Check sheet for the drawn part. Datum: minimum x, y, z corner. Units: mm. A direction names the side the tool comes from. Round coordinates to 2 decimals unless told otherwise and drop trailing zeros. Write each loop counter-clockwise with the first axis right and the second up, starting at its lowest first coordinate (ties: lowest second). Pieces come first, ordered by that corner, then holes. Notation, with made-up numbers: (56.5, 82) - (69.5, 82) arc R12 ccw to (69.5, 88) - close; hole circle Ø7 at (0.5, -39.5). An arc over 180 degrees is marked (long way). Return JSON: item names as keys, results as strings. Group by question number.
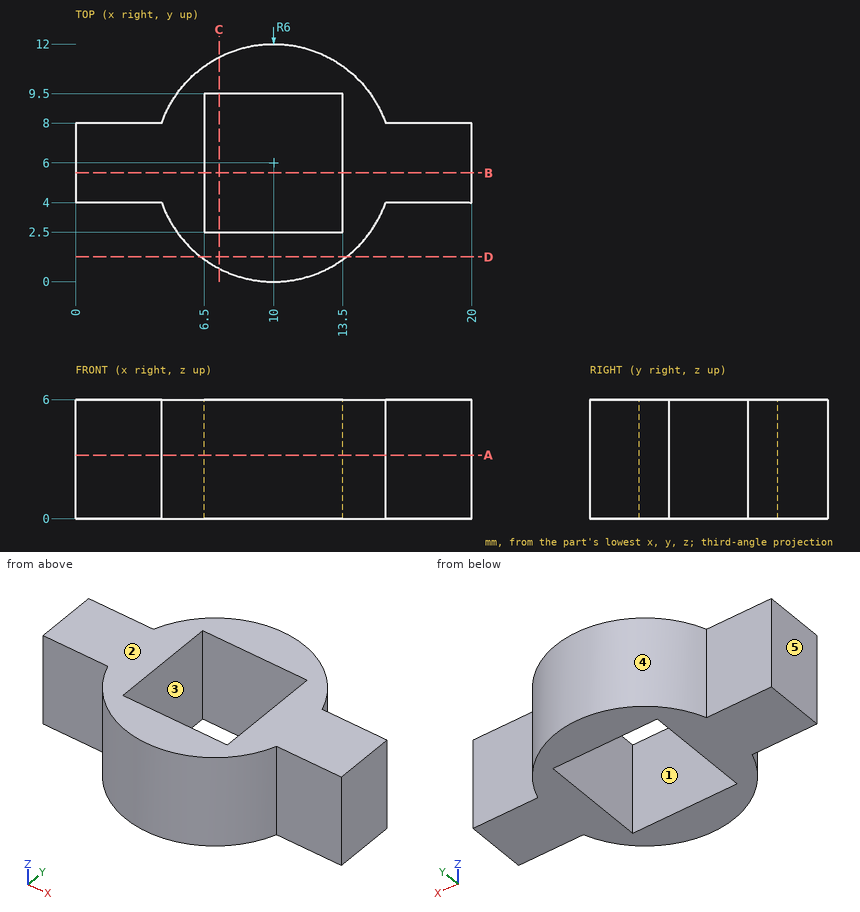
1. Section check A-A (z = 3.2). Enter the section's corners in (x, y).
2. Tool access check on the marked faces 1 and 2. Record the directions out of +Z, -Z, +X, -X, +Y, -Y that give a thin tool (end or side, any length) a straight path to the whole face; none if there is none.
3. Depth check by flat-ended pin: pin 1 Ø3 at (x, z) = (8, 5.5) entering from +Y; pin 2 Ø3.5 at (x, z) = (3, 1.5) entering from -Y; pin 3 Ø2 at (x, z) = (18, 2) entering from +Y; pin 4 Ø6 at (x, y) = (8.5, 2.5) entering from -Z. Enter the tip coordinate at first touch or a pass-through.
4. Section check C-C (x = 7.25). Enter the section's corners in (y, z).
5. Material ranges on line 1 along X through (y, z) = (5.25, 0.45); line 2 along Y through (x, z) = (10, 1.55); line 3 along X through (y, z) = (3.5, 3.4), recorded low to high.
6. Mould release check, pull along X, two halves, no side actions. Record for the marked faces 3, 4 and 5: pulls with the +X half, pulls with the -X half, needs draft (parallel to the pull), parting line crosses it, or undercut.
7. Section check D-D (y = 1.25). Enter the section's corners in (x, z).
8. Section check B-B (y = 5.5). Enter the section's corners in (x, z), and give its area (3 significant figures).
Result sheet:
{
 "1": {"outline": "(0, 4) - (4.34, 4) arc R6 ccw to (15.66, 4) - (20, 4) - (20, 8) - (15.66, 8) arc R6 ccw to (4.34, 8) - (0, 8) - close; hole (6.5, 2.5) - (13.5, 2.5) - (13.5, 9.5) - (6.5, 9.5) - close"},
 "2": {"face 1": "+Z, -Z", "face 2": "+Z, +X, -X, +Y, -Y"},
 "3": {"pin 1": "stops at y = 11.98", "pin 2": "stops at y = 3.1", "pin 3": "stops at y = 8", "pin 4": "stops at z = 0"},
 "4": {"outline": "(0.67, 0) - (2.5, 0) - (2.5, 6) - (0.67, 6) - close; (9.5, 0) - (11.33, 0) - (11.33, 6) - (9.5, 6) - close"},
 "5": {"line 1": "x = 0 to 6.5, 13.5 to 20", "line 2": "y = 0 to 2.5, 9.5 to 12", "line 3": "x = 4.55 to 6.5, 13.5 to 15.45"},
 "6": {"face 3": "undercut", "face 4": "parting line crosses it", "face 5": "pulls with the -X half"},
 "7": {"outline": "(6.33, 0) - (13.67, 0) - (13.67, 6) - (6.33, 6) - close"},
 "8": {"outline": "(0, 0) - (6.5, 0) - (6.5, 6) - (0, 6) - close; (13.5, 0) - (20, 0) - (20, 6) - (13.5, 6) - close", "area": "78.0 mm²"}
}
